Verification items for this drawing (mm, ordinates from the low corner). Coordinates: 2 decimals unless noted, no trailing zeros. Write each loop counter-clockwise with the first axis right and the second up, starting at its lowest first coordinate (ties: lowest second). Pieces come first, ordered by that corner, then holes. Notation, with made-up numbers: (-38, -39) -> (-11, -39) arc R26 cw to (-11, -16) -> close; hole circle Ø8 at (15, 77). An arc over 180 degrees is marked (long way). Answer as CSV lines item,"result".
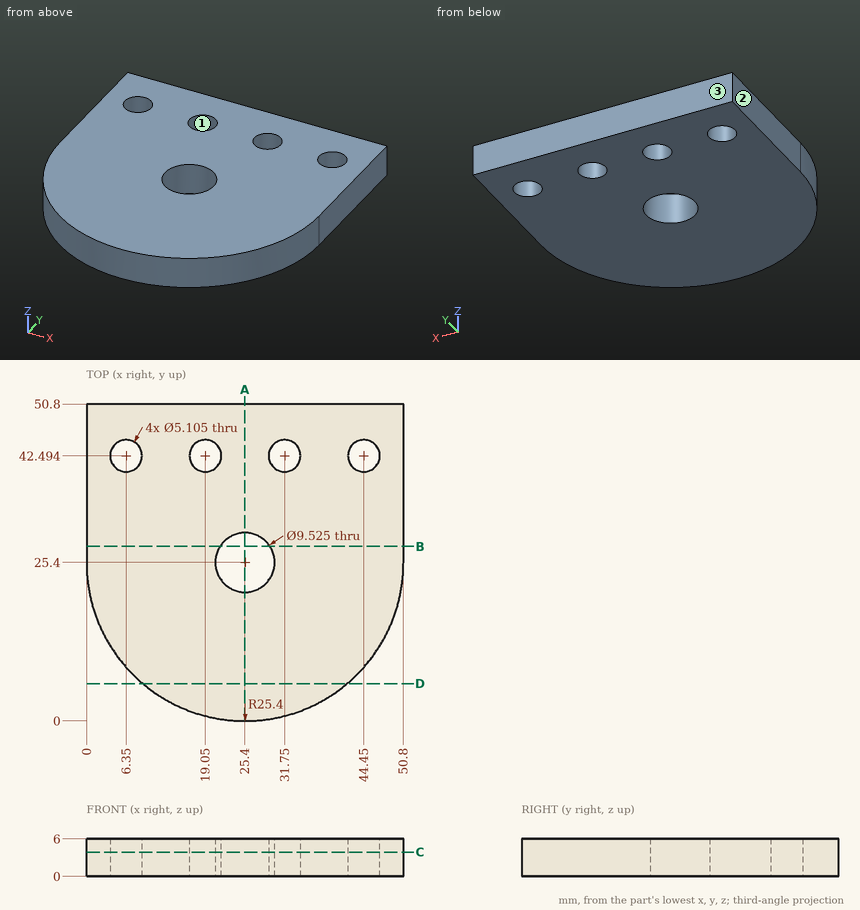
Item 1: Thickness scan on probe 1 along Y at (x, z) = (6.35, 2.85) (1 decimal); probe 2 along Y at (x, z) = (45, 4.85) (1 decimal); probe 3 along X at (y, z) = (44, 4.5). Record the ranges inside material, lowest first.
Responses:
probe 1,"y = 8.6 to 39.9, 45 to 50.8"
probe 2,"y = 9.2 to 40, 45 to 50.8"
probe 3,"x = 0 to 4.29, 8.41 to 16.99, 21.11 to 29.69, 33.81 to 42.39, 46.51 to 50.8"
Item 2: Cross-section at D-D, the plane y = 6. Record the cut outline in (x, z) (1 decimal).
Responses:
outline,"(9, 0) -> (41.8, 0) -> (41.8, 6) -> (9, 6) -> close"
Item 3: Cross-section at A-A, the plane x = 25.4. Record the cut outline in (y, z), plus the area to 3 significant figures.
Responses:
outline,"(0, 0) -> (20.64, 0) -> (20.64, 6) -> (0, 6) -> close; (30.16, 0) -> (50.8, 0) -> (50.8, 6) -> (30.16, 6) -> close"
area,"248 mm2"
Item 4: Cross-section at B-B, the plane y = 28. Record the cut outline in (x, z).
Responses:
outline,"(0, 0) -> (21.41, 0) -> (21.41, 6) -> (0, 6) -> close; (29.39, 0) -> (50.8, 0) -> (50.8, 6) -> (29.39, 6) -> close"
Item 5: Release check for a two-part mould opening along Y. For the marked faces 1, 2 and 3 record: +Y half, -Y half, draft (parallel to the pull), parting line (faces both ways), or undercut.
Responses:
face 1,"undercut"
face 2,"draft"
face 3,"+Y half"
Item 6: Depth check by flat-ended pin: pin 1 Ø3 at (y, z) = (9.5, 4.5) entering from -X; pin 2 Ø6.5 at (x, y) = (44.45, 42.49) entering from -Z; pin 3 Ø2 at (x, z) = (30, 1.5) entering from -Y; pin 4 Ø4.5 at (x, y) = (31.75, 42.49) entering from -Z. Enter the tip coordinate at first touch or a pass-through.
Responses:
pin 1,"stops at x = 4.48"
pin 2,"stops at z = 0"
pin 3,"stops at y = 0.26"
pin 4,"passes through"
Item 7: Cross-section at C-C, the plane z = 3.9. Count the separate pieces of the cut face and the enclosed holes in it, plus the area to 3 significant figures.
Responses:
separate pieces,"1"
enclosed holes,"5"
area,"2,150 mm2"
